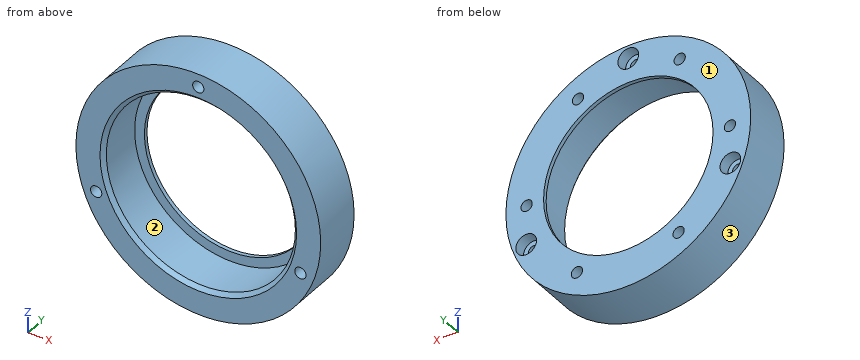
from build123d import *

# Parameters (mm, degrees)
SKETCH1_R           = 32.5
SKETCH1_R_2         = 25.1
BOSS_EXTRUDE1_DEPTH = 13
SKETCH2_R           = 25.1
SKETCH2_R_2         = 22.5
BOSS_EXTRUDE2_DEPTH = 1
SKETCH3_R           = 1.5
CUT_EXTRUDE1_DEPTH  = 14
CHAMFER1_SIZE       = 1
SKETCH4_R           = 2.75
CUT_EXTRUDE2_DEPTH  = 3
SKETCH5_R           = 1.5
CUT_EXTRUDE3_DEPTH  = 10


with BuildPart() as part:
    # Sketch1 → Boss-Extrude1 (new body)
    with BuildSketch(Plane(origin=(0, 0, 0), x_dir=(1, 0, 0), z_dir=(0, 1, 0))):
        Circle(SKETCH1_R)
        Circle(SKETCH1_R_2, mode=Mode.SUBTRACT)
    extrude(amount=BOSS_EXTRUDE1_DEPTH)

    # Sketch2 → Boss-Extrude2 (add)
    with BuildSketch(Plane(origin=(0, 13, 0), x_dir=(1, 0, 0), z_dir=(0, 1, 0))):
        Circle(SKETCH2_R)
        Circle(SKETCH2_R_2, mode=Mode.SUBTRACT)
    extrude(amount=-BOSS_EXTRUDE2_DEPTH)

    # Sketch3 → Cut-Extrude1 (cut, through all)
    with BuildSketch(Plane(origin=(0, 0, 0), x_dir=(-1, 0, 0), z_dir=(0, -1, 0))):
        with Locations((0, -29)):
            Circle(SKETCH3_R)
        with Locations((-27.115332973, 10.283905765)):
            Circle(SKETCH3_R)
        with Locations((27.115332973, 10.283905765)):
            Circle(SKETCH3_R)
    extrude(amount=-CUT_EXTRUDE1_DEPTH, mode=Mode.SUBTRACT)

    # Chamfer1
    chamfer1_edges = [part.edges().sort_by_distance(p)[0] for p in [
        (-25.1, 0, 0),
    ]]
    chamfer(chamfer1_edges, length=CHAMFER1_SIZE)

    # Sketch4 → Cut-Extrude2 (cut)
    with BuildSketch(Plane(origin=(0, 13, 0), x_dir=(1, 0, 0), z_dir=(0, 1, 0))):
        with Locations((-27.115332973, 10.283905765)):
            Circle(SKETCH4_R)
        with Locations((27.115332973, 10.283905765)):
            Circle(SKETCH4_R)
        with Locations((0, -29)):
            Circle(SKETCH4_R)
    extrude(amount=-CUT_EXTRUDE2_DEPTH, mode=Mode.SUBTRACT)

    # Sketch5 → Cut-Extrude3 (cut)
    with BuildSketch(Plane(origin=(0, 13, 0), x_dir=(1, 0, 0), z_dir=(0, 1, 0))):
        with Locations((13.641823983, 23.300228291)):
            Circle(SKETCH5_R)
        with Locations((26.999501606, -0.164051977)):
            Circle(SKETCH5_R)
        with Locations((13.357677623, -23.464280269)):
            Circle(SKETCH5_R)
        with Locations((-13.641823983, -23.300228291)):
            Circle(SKETCH5_R)
        with Locations((-26.999501606, 0.164051977)):
            Circle(SKETCH5_R)
        with Locations((-13.357677623, 23.464280269)):
            Circle(SKETCH5_R)
    extrude(amount=-CUT_EXTRUDE3_DEPTH, mode=Mode.SUBTRACT)


solid = part.part
Geometry check sheet. Reference: the model listing, model coordinates, mm. Face numbers are marked on the shaded views. Round coordinates to 2 decimals unless told otherwise and drop trailing zeros. Loops run counter-clockwise (first coordinate to the right, second up) from the corner with the lowest first, then second, coordinate; pieces in that order, holes last.
Item 1: Cross-section at C-C on y = 11. Count the separate pieces of the cut face and the enclosed holes in it, then the cut area to 3 significant figures.
Item 2: Gauge pin test, flat ends, axial feed: pin 1 (4 mm diameter, centred on y = 7, z = 3.5, fed in from -X); pin 2 (2.5 mm diameter, centred on x = 27.12, z = -10.28, fed in from -Y) (3 decimals); pin 3 (5 mm diameter, centred on y = 2.5, z = -12, fed in from -X); pin 4 (3 mm diameter, centred on x = -28, z = -10, fed in from +Y). Record the tip position at first contact, or that the pin passes through.
Item 3: Mould release check, pull along Z, two halves, no side actions. Record for the marked faces 1, 2 and 3: pulls with the +Z half, pulls with the -Z half, needs draft (parallel to the pull), parting line crosses it, or undercut.
Item 4: Cross-section at A-A on x = 0. Record the boundary of the cut face in (y, z), then the cut area to 3 significant figures.
Item 5: Cross-section at B-B on z = 29. Record the boundary of the cut face in (x, y), then the cut area to 3 significant figures.
Item 6: Thickness scan on line 1 (Z direction, x = 0, y = 8.25); line 2 (X direction, y = 12.4, z = 0); line 3 (Z direction, x = 13.5, y = 8.25). Record the ranges inside material, lowest first.
Answer sheet:
1. separate pieces: 1
1. enclosed holes: 10
1. area: 1,230 mm2
2. pin 1: stops at x = -32.47
2. pin 2: passes through
2. pin 3: stops at x = -31.08
2. pin 4: stops at y = 10
3. face 1: needs draft
3. face 2: undercut
3. face 3: parting line crosses it
4. outline: (0, -32.5) - (13, -32.5) - (13, -22.5) - (12, -22.5) - (12, -25.1) - (1, -25.1) - (0, -26.1) - close; (0, 26.1) - (1, 25.1) - (12, 25.1) - (12, 22.5) - (13, 22.5) - (13, 26.25) - (10, 26.25) - (10, 27.5) - (0, 27.5) - close; (0, 30.5) - (10, 30.5) - (10, 31.75) - (13, 31.75) - (13, 32.5) - (0, 32.5) - close
4. area: 150 mm2
5. outline: (-14.67, 0) - (-1.5, 0) - (-1.5, 10) - (-2.75, 10) - (-2.75, 13) - (-14.67, 13) - close; (1.5, 0) - (14.67, 0) - (14.67, 13) - (2.75, 13) - (2.75, 10) - (1.5, 10) - close
5. area: 335 mm2
6. line 1: z = -32.5 to -25.1, 25.1 to 27.5, 30.5 to 32.5
6. line 2: x = -32.5 to -28.49, -25.51 to -22.5, 22.5 to 25.51, 28.49 to 32.5
6. line 3: z = -29.56 to -24.79, -21.81 to -21.16, 21.16 to 21.97, 24.96 to 29.56
